```python
from build123d import *

# Parameters (mm, degrees)
F0_W     = 131.982717663
F0_H     = 104.5415252447
F0_W_2   = 119.2827182055
F0_H_2   = 91.8415257871
F1_DEPTH = 127
F2_DEPTH = 50.8


with BuildPart() as f1:
    # F0 (on Front) → F1 (new body, symmetric)
    with BuildSketch(Plane.XZ):
        with Locations((7.0537086576, -15.5196636915)):
            Rectangle(F0_W, F0_H)
        with Locations((7.0537083864, -15.5196639627)):
            Rectangle(F0_W_2, F0_H_2, mode=Mode.SUBTRACT)
    extrude(amount=F1_DEPTH, both=True)

    # F2 (add): a face of the model
    f2_faces = [f1.faces().sort_by_distance(p)[0] for p in [
        (7.0537083864, 0, 30.4010989308),
    ]]
    extrude(f2_faces, amount=F2_DEPTH)


solid = f1.part
```
The listing builds one solid part. Answer for the finished solid, in the listing's coordinates (mm). A direction names the side the tool comes from. Coordinates: 2 decimals unless noted, no trailing zeros. Loops run counter-clockwise (first coordinate to the right, second up) from the corner with the lowest first, then second, coordinate; pieces in that order, holes last. Notation, with made-up numbers: (35, 23) - (70, 23) arc R17 cw to (70, 55) - close; hole circle Ø9 at (89, -13). An arc over 180 degrees is marked (long way). Write item = value, one per line.
1) Determine the mould class of faces 3 (the face through (6, -2, -61.44)), 4 (the face through (6, -2, -67.79)), 5 (the face through (73.045, -2, -16)), 6 (the face through (-58.938, -2, -16)) for opening direction X: pulls with the +X half, pulls with the -X half, needs draft (parallel to the pull), parting line crosses it, or undercut.
Responses:
face_3 = undercut
face_4 = needs draft
face_5 = pulls with the +X half
face_6 = pulls with the -X half
2) Which of the six approach directions +Z, -Z, +X, -X, +Y, -Y give full straight-line access (tool end or side, diameter ignored) to faces 1 (the face through (6, -2, -20.399)), 2 (the face through (6, 127, 8))?
Responses:
face_1 = +Y, -Y
face_2 = +Z, -Z, +X, -X, +Y
3) Section B-B (z = -39) is taken. Determine the outline of the cut face in (x, y), plus the area to 3 significant figures.
Responses:
outline = (-58.94, -127) - (-52.59, -127) - (-52.59, 127) - (-58.94, 127) - close; (66.7, -127) - (73.05, -127) - (73.05, 127) - (66.7, 127) - close
area = 3,230 mm^2
4) Section C-C (y = -6.5) is taken. Determine the outline of the cut face in (x, z), plus the area to 3 significant figures.
Responses:
outline = (-58.94, -67.79) - (73.05, -67.79) - (73.05, 36.75) - (-58.94, 36.75) - close; hole (-52.59, -61.44) - (66.7, -61.44) - (66.7, -20.4) - (-52.59, -20.4) - close
area = 8,900 mm^2
5) Find the intervals of material crossed by line 1 along Z through (x, y) = (39, 36); line 2 along X through (y, z) = (-17.5, -57), in increasing order.
Responses:
line_1 = -67.79 to -61.44, -20.4 to 36.75
line_2 = -58.94 to -52.59, 66.7 to 73.05
6) Section A-A (x = 30) is taken. Determine the outline of the cut face in (y, z).
Responses:
outline = (-127, -67.79) - (127, -67.79) - (127, -61.44) - (-127, -61.44) - close; (-127, -20.4) - (127, -20.4) - (127, 36.75) - (-127, 36.75) - close
